from build123d import *

# Parameters (mm, degrees)
RESSALTO_EXTRUS_O2_DEPTH = 13
ESBO_O3_R                = 1.5
CORTE_EXTRUS_O2_DEPTH    = 13


with BuildPart() as part:
    # Esboço1 → Ressalto-extrusão2 (new body)
    with BuildSketch(Plane.XY):
        Polygon((-7.457901998, 2.385917031), (-7.230517524, 2.385917031), (4.042098002, 2.385917031), (10.042098002, 2.385917031), (10.042098002, 5.385917031), (-13.457901998, 5.385917031), (-13.457901998, 2.385917031), align=None)
    extrude(amount=RESSALTO_EXTRUS_O2_DEPTH)

    # Esboço3 → Corte-extrusão2 (cut)
    with BuildSketch(Plane(origin=(0, 5.385917031, 0), x_dir=(1, 0, 0), z_dir=(0, 1, 0))):
        with Locations(Location((-1.707901998, -6, 0), (0, 0, 180))):
            Circle(ESBO_O3_R)
    extrude(amount=-CORTE_EXTRUS_O2_DEPTH, mode=Mode.SUBTRACT)


solid = part.part
Geometry check sheet. Reference: the model listing, model coordinates, mm. Give positions to 0.01 mm unless a question says otherwise; leave off trailing zeros. Write each loop counter-clockwise with the first axis right and the second up, starting at its lowest first coordinate (ties: lowest second). Pieces come first, ordered by that corner, then holes.
1) Cross-section at A-A (z = 6). Record the boundary of the cut face in (x, y), plus the area to 3 significant figures.
Values follow:
outline: (-13.46, 2.39) - (-3.21, 2.39) - (-3.21, 5.39) - (-13.46, 5.39) - close; (-0.21, 2.39) - (10.04, 2.39) - (10.04, 5.39) - (-0.21, 5.39) - close
area: 61.5 mm2
2) Cross-section at B-B (x = -2). Record the boundary of the cut face in (y, z), plus the area to 3 significant figures.
Values follow:
outline: (2.39, 0) - (5.39, 0) - (5.39, 4.53) - (2.39, 4.53) - close; (2.39, 7.47) - (5.39, 7.47) - (5.39, 13) - (2.39, 13) - close
area: 30.2 mm2
3) Thickness scan on line 1 (Z direction, x = -2.25, y = 4.2); line 2 (X direction, y = 4.05, z = 5.5); line 3 (X direction, y = 5, z = 6.75). Record the ranges inside material, lowest first.
Values follow:
line 1: z = 0 to 4.6, 7.4 to 13
line 2: x = -13.46 to -3.12, -0.29 to 10.04
line 3: x = -13.46 to -3.01, -0.41 to 10.04
4) Cross-section at C-C (y = 3.7). Record the boundary of the cut face in (x, z).
Values follow:
outline: (-13.46, 0) - (10.04, 0) - (10.04, 13) - (-13.46, 13) - close; hole circle Ø3 at (-1.71, 6)
